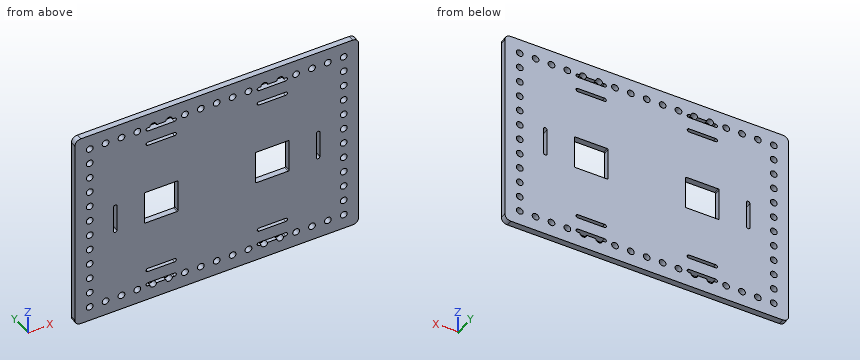
```python
from build123d import *

# Parameters (mm, degrees)
SKETCH1_R           = 1.7
BOSS_EXTRUDE1_DEPTH = 3


with BuildPart() as part:
    # Sketch1 → Boss-Extrude1 (new body)
    with BuildSketch(Plane(origin=(0, 3, 0), x_dir=(1, 0, 0), z_dir=(0, 1, 0))):
        with BuildLine():
            Line((71.5, -48.5), (71.5, 48.5))
            ThreePointArc((71.5, 48.5), (70.621320344, 50.621320344), (68.5, 51.5))
            Line((68.5, 51.5), (-68.5, 51.5))
            ThreePointArc((-68.5, 51.5), (-70.621320344, 50.621320344), (-71.5, 48.5))
            Line((-71.5, 48.5), (-71.5, -48.5))
            ThreePointArc((-71.5, -48.5), (-70.621320344, -50.621320344), (-68.5, -51.5))
            Line((-68.5, -51.5), (68.5, -51.5))
            ThreePointArc((68.5, -51.5), (70.621320344, -50.621320344), (71.5, -48.5))
        make_face()
        with Locations(Location((-64, 44, 0), (0, 0, 90))):
            Circle(SKETCH1_R, mode=Mode.SUBTRACT)
        with Locations(Location((-64, 28, 0), (0, 0, 90))):
            Circle(SKETCH1_R, mode=Mode.SUBTRACT)
        with Locations(Location((-64, 12, 0), (0, 0, 90))):
            Circle(SKETCH1_R, mode=Mode.SUBTRACT)
        with Locations(Location((-64, -4, 0), (0, 0, 90))):
            Circle(SKETCH1_R, mode=Mode.SUBTRACT)
        with Locations(Location((-64, -20, 0), (0, 0, 90))):
            Circle(SKETCH1_R, mode=Mode.SUBTRACT)
        with Locations(Location((-64, -36, 0), (0, 0, 90))):
            Circle(SKETCH1_R, mode=Mode.SUBTRACT)
        with Locations(Location((56, -44, 0), (0, 0, 90))):
            Circle(SKETCH1_R, mode=Mode.SUBTRACT)
        with Locations(Location((40, -44, 0), (0, 0, 90))):
            Circle(SKETCH1_R, mode=Mode.SUBTRACT)
        with Locations(Location((8, -44, 0), (0, 0, 90))):
            Circle(SKETCH1_R, mode=Mode.SUBTRACT)
        with Locations(Location((-8, -44, 0), (0, 0, 90))):
            Circle(SKETCH1_R, mode=Mode.SUBTRACT)
        with Locations(Location((-40, -44, 0), (0, 0, 90))):
            Circle(SKETCH1_R, mode=Mode.SUBTRACT)
        with Locations(Location((-56, -44, 0), (0, 0, 90))):
            Circle(SKETCH1_R, mode=Mode.SUBTRACT)
        with Locations(Location((-64, -44, 0), (0, 0, 90))):
            Circle(SKETCH1_R, mode=Mode.SUBTRACT)
        with Locations(Location((-48, -44, 0), (0, 0, 90))):
            Circle(SKETCH1_R, mode=Mode.SUBTRACT)
        with Locations(Location((-16, -44, 0), (0, 0, 90))):
            Circle(SKETCH1_R, mode=Mode.SUBTRACT)
        with Locations(Location((0, -44, 0), (0, 0, 90))):
            Circle(SKETCH1_R, mode=Mode.SUBTRACT)
        with Locations(Location((16, -44, 0), (0, 0, 90))):
            Circle(SKETCH1_R, mode=Mode.SUBTRACT)
        with Locations(Location((48, -44, 0), (0, 0, 90))):
            Circle(SKETCH1_R, mode=Mode.SUBTRACT)
        with Locations(Location((64, -44, 0), (0, 0, 90))):
            Circle(SKETCH1_R, mode=Mode.SUBTRACT)
        with Locations(Location((-64, -28, 0), (0, 0, 90))):
            Circle(SKETCH1_R, mode=Mode.SUBTRACT)
        with Locations(Location((-64, -12, 0), (0, 0, 90))):
            Circle(SKETCH1_R, mode=Mode.SUBTRACT)
        with Locations(Location((-64, 4, 0), (0, 0, 90))):
            Circle(SKETCH1_R, mode=Mode.SUBTRACT)
        with Locations(Location((-64, 20, 0), (0, 0, 90))):
            Circle(SKETCH1_R, mode=Mode.SUBTRACT)
        with Locations(Location((-64, 36, 0), (0, 0, 90))):
            Circle(SKETCH1_R, mode=Mode.SUBTRACT)
        with Locations(Location((64, -20, 0), (0, 0, 90))):
            Circle(SKETCH1_R, mode=Mode.SUBTRACT)
        with Locations(Location((64, -4, 0), (0, 0, 90))):
            Circle(SKETCH1_R, mode=Mode.SUBTRACT)
        with Locations(Location((64, 12, 0), (0, 0, 90))):
            Circle(SKETCH1_R, mode=Mode.SUBTRACT)
        with Locations(Location((64, 28, 0), (0, 0, 90))):
            Circle(SKETCH1_R, mode=Mode.SUBTRACT)
        with Locations(Location((-48, 44, 0), (0, 0, 90))):
            Circle(SKETCH1_R, mode=Mode.SUBTRACT)
        with Locations(Location((-16, 44, 0), (0, 0, 90))):
            Circle(SKETCH1_R, mode=Mode.SUBTRACT)
        with Locations(Location((0, 44, 0), (0, 0, 90))):
            Circle(SKETCH1_R, mode=Mode.SUBTRACT)
        with Locations(Location((16, 44, 0), (0, 0, 90))):
            Circle(SKETCH1_R, mode=Mode.SUBTRACT)
        with Locations(Location((48, 44, 0), (0, 0, 90))):
            Circle(SKETCH1_R, mode=Mode.SUBTRACT)
        with Locations(Location((64, 44, 0), (0, 0, 90))):
            Circle(SKETCH1_R, mode=Mode.SUBTRACT)
        with Locations(Location((56, 44, 0), (0, 0, 90))):
            Circle(SKETCH1_R, mode=Mode.SUBTRACT)
        with Locations(Location((40, 44, 0), (0, 0, 90))):
            Circle(SKETCH1_R, mode=Mode.SUBTRACT)
        with Locations(Location((8, 44, 0), (0, 0, 90))):
            Circle(SKETCH1_R, mode=Mode.SUBTRACT)
        with Locations(Location((-8, 44, 0), (0, 0, 90))):
            Circle(SKETCH1_R, mode=Mode.SUBTRACT)
        with Locations(Location((-40, 44, 0), (0, 0, 90))):
            Circle(SKETCH1_R, mode=Mode.SUBTRACT)
        with Locations(Location((-56, 44, 0), (0, 0, 90))):
            Circle(SKETCH1_R, mode=Mode.SUBTRACT)
        with Locations(Location((64, 36, 0), (0, 0, 90))):
            Circle(SKETCH1_R, mode=Mode.SUBTRACT)
        with Locations(Location((64, 20, 0), (0, 0, 90))):
            Circle(SKETCH1_R, mode=Mode.SUBTRACT)
        with Locations(Location((64, 4, 0), (0, 0, 90))):
            Circle(SKETCH1_R, mode=Mode.SUBTRACT)
        with Locations(Location((64, -12, 0), (0, 0, 90))):
            Circle(SKETCH1_R, mode=Mode.SUBTRACT)
        with Locations(Location((64, -28, 0), (0, 0, 90))):
            Circle(SKETCH1_R, mode=Mode.SUBTRACT)
        with Locations(Location((64, -36, 0), (0, 0, 90))):
            Circle(SKETCH1_R, mode=Mode.SUBTRACT)
        with BuildLine():
            Line((21.25, 44.05), (22.300735453, 44.05))
            ThreePointArc((22.300735453, 44.05), (24, 45.7), (25.699264547, 44.05))
            Line((25.699264547, 44.05), (30.300735453, 44.05))
            ThreePointArc((30.300735453, 44.05), (32, 45.7), (33.699264547, 44.05))
            Line((33.699264547, 44.05), (34.75, 44.05))
            ThreePointArc((34.75, 44.05), (35.625, 43.175), (34.75, 42.3))
            Line((34.75, 42.3), (21.25, 42.3))
            ThreePointArc((21.25, 42.3), (20.375, 43.175), (21.25, 44.05))
        make_face(mode=Mode.SUBTRACT)
        with BuildLine():
            Line((22.300735453, -44.05), (21.25, -44.05))
            ThreePointArc((21.25, -44.05), (20.375, -43.175), (21.25, -42.3))
            Line((21.25, -42.3), (34.75, -42.3))
            ThreePointArc((34.75, -42.3), (35.625, -43.175), (34.75, -44.05))
            Line((34.75, -44.05), (33.699264547, -44.05))
            ThreePointArc((33.699264547, -44.05), (32, -45.7), (30.300735453, -44.05))
            Line((30.300735453, -44.05), (25.699264547, -44.05))
            ThreePointArc((25.699264547, -44.05), (24, -45.7), (22.300735453, -44.05))
        make_face(mode=Mode.SUBTRACT)
        with BuildLine():
            Line((21.25, 36.05), (34.75, 36.05))
            ThreePointArc((34.75, 36.05), (35.625, 35.175), (34.75, 34.3))
            Line((34.75, 34.3), (21.25, 34.3))
            ThreePointArc((21.25, 34.3), (20.375, 35.175), (21.25, 36.05))
        make_face(mode=Mode.SUBTRACT)
        with BuildLine():
            Line((50.25, -6.75), (50.25, 6.75))
            ThreePointArc((50.25, 6.75), (51.125, 7.625), (52, 6.75))
            Line((52, 6.75), (52, -6.75))
            ThreePointArc((52, -6.75), (51.125, -7.625), (50.25, -6.75))
        make_face(mode=Mode.SUBTRACT)
        with BuildLine():
            Line((21.25, -34.3), (34.75, -34.3))
            ThreePointArc((34.75, -34.3), (35.625, -35.175), (34.75, -36.05))
            Line((34.75, -36.05), (21.25, -36.05))
            ThreePointArc((21.25, -36.05), (20.375, -35.175), (21.25, -34.3))
        make_face(mode=Mode.SUBTRACT)
        with BuildLine():
            Line((36, -8.5), (20, -8.5))
            ThreePointArc((20, -8.5), (19.646446609, -8.353553391), (19.5, -8))
            Line((19.5, -8), (19.5, 8))
            ThreePointArc((19.5, 8), (19.646446609, 8.353553391), (20, 8.5))
            Line((20, 8.5), (36, 8.5))
            ThreePointArc((36, 8.5), (36.353553391, 8.353553391), (36.5, 8))
            Line((36.5, 8), (36.5, -8))
            ThreePointArc((36.5, -8), (36.353553391, -8.353553391), (36, -8.5))
        make_face(mode=Mode.SUBTRACT)
        with BuildLine():
            Line((-21.25, 34.3), (-34.75, 34.3))
            ThreePointArc((-34.75, 34.3), (-35.625, 35.175), (-34.75, 36.05))
            Line((-34.75, 36.05), (-21.25, 36.05))
            ThreePointArc((-21.25, 36.05), (-20.375, 35.175), (-21.25, 34.3))
        make_face(mode=Mode.SUBTRACT)
        with BuildLine():
            Line((-50.25, 6.75), (-50.25, -6.75))
            ThreePointArc((-50.25, -6.75), (-51.125, -7.625), (-52, -6.75))
            Line((-52, -6.75), (-52, 6.75))
            ThreePointArc((-52, 6.75), (-51.125, 7.625), (-50.25, 6.75))
        make_face(mode=Mode.SUBTRACT)
        with BuildLine():
            Line((-21.25, -36.05), (-34.75, -36.05))
            ThreePointArc((-34.75, -36.05), (-35.625, -35.175), (-34.75, -34.3))
            Line((-34.75, -34.3), (-21.25, -34.3))
            ThreePointArc((-21.25, -34.3), (-20.375, -35.175), (-21.25, -36.05))
        make_face(mode=Mode.SUBTRACT)
        with BuildLine():
            Line((-19.5, 8), (-19.5, -8))
            ThreePointArc((-19.5, -8), (-19.646446609, -8.353553391), (-20, -8.5))
            Line((-20, -8.5), (-36, -8.5))
            ThreePointArc((-36, -8.5), (-36.353553391, -8.353553391), (-36.5, -8))
            Line((-36.5, -8), (-36.5, 8))
            ThreePointArc((-36.5, 8), (-36.353553391, 8.353553391), (-36, 8.5))
            Line((-36, 8.5), (-20, 8.5))
            ThreePointArc((-20, 8.5), (-19.646446609, 8.353553391), (-19.5, 8))
        make_face(mode=Mode.SUBTRACT)
        with BuildLine():
            Line((-34.75, -42.3), (-21.25, -42.3))
            ThreePointArc((-21.25, -42.3), (-20.375, -43.175), (-21.25, -44.05))
            Line((-21.25, -44.05), (-22.300735453, -44.05))
            ThreePointArc((-22.300735453, -44.05), (-24, -45.7), (-25.699264547, -44.05))
            Line((-25.699264547, -44.05), (-30.300735453, -44.05))
            ThreePointArc((-30.300735453, -44.05), (-32, -45.7), (-33.699264547, -44.05))
            Line((-33.699264547, -44.05), (-34.75, -44.05))
            ThreePointArc((-34.75, -44.05), (-35.625, -43.175), (-34.75, -42.3))
        make_face(mode=Mode.SUBTRACT)
        with BuildLine():
            Line((-34.75, 44.05), (-33.699264547, 44.05))
            ThreePointArc((-33.699264547, 44.05), (-32, 45.7), (-30.300735453, 44.05))
            Line((-30.300735453, 44.05), (-25.699264547, 44.05))
            ThreePointArc((-25.699264547, 44.05), (-24, 45.7), (-22.300735453, 44.05))
            Line((-22.300735453, 44.05), (-21.25, 44.05))
            ThreePointArc((-21.25, 44.05), (-20.375, 43.175), (-21.25, 42.3))
            Line((-21.25, 42.3), (-34.75, 42.3))
            ThreePointArc((-34.75, 42.3), (-35.625, 43.175), (-34.75, 44.05))
        make_face(mode=Mode.SUBTRACT)
    extrude(amount=-BOSS_EXTRUDE1_DEPTH)


solid = part.part
```
Build history of the part. All positions in model axes, mm. Give positions to 0.01 mm unless a question says otherwise; leave off trailing zeros. Loops run counter-clockwise (first coordinate to the right, second up) from the corner with the lowest first, then second, coordinate; pieces in that order, holes last.
1) Drop a flat-ended pin along its axis: P1, Ø4.5, axis at x = -48, z = -44, coming from the -Y side. Give the stop position or say it passes through.
Values follow:
P1: stops at y = 0
2) Probe line 1 along X through (y, z) = (0.7, -12); line 2 along Z through (x, y) = (-48, 2.35); line 3 along Z through (x, y) = (30, 1.95). List the from-to ranges inside material, lowest first.
Values follow:
line 1: x = -71.5 to -65.7, -62.3 to 62.3, 65.7 to 71.5
line 2: z = -51.5 to -45.7, -42.3 to 42.3, 45.7 to 51.5
line 3: z = -51.5 to -44.05, -42.3 to -36.05, -34.3 to -8.5, 8.5 to 34.3, 36.05 to 42.3, 44.05 to 51.5
3) Band-saw the part on D-D on x = -64. State how many separate pieces and enclosed holes the cut face has, then the cut area to 3 significant figures.
Values follow:
separate pieces: 13
enclosed holes: 0
area: 187 mm2
4) Band-saw the part on C-C on x = -32. List the corners of the cut face in (y, z), then the cut area to 3 significant figures.
Values follow:
outline: (0, -51.5) - (3, -51.5) - (3, -45.7) - (0, -45.7) - close; (0, -42.3) - (3, -42.3) - (3, -36.05) - (0, -36.05) - close; (0, -34.3) - (3, -34.3) - (3, -8.5) - (0, -8.5) - close; (0, 8.5) - (3, 8.5) - (3, 34.3) - (0, 34.3) - close; (0, 36.05) - (3, 36.05) - (3, 42.3) - (0, 42.3) - close; (0, 45.7) - (3, 45.7) - (3, 51.5) - (0, 51.5) - close
area: 227 mm2
5) Band-saw the part on B-B on z = -20. List the corners of the cut face in (x, y), then the cut area to 3 significant figures.
Values follow:
outline: (-71.5, 0) - (-65.7, 0) - (-65.7, 3) - (-71.5, 3) - close; (-62.3, 0) - (62.3, 0) - (62.3, 3) - (-62.3, 3) - close; (65.7, 0) - (71.5, 0) - (71.5, 3) - (65.7, 3) - close
area: 409 mm2
6) Band-saw the part on A-A on x = -8. List the corners of the cut face in (y, z), then the cut area to 3 significant figures.
Values follow:
outline: (0, -51.5) - (3, -51.5) - (3, -45.7) - (0, -45.7) - close; (0, -42.3) - (3, -42.3) - (3, 42.3) - (0, 42.3) - close; (0, 45.7) - (3, 45.7) - (3, 51.5) - (0, 51.5) - close
area: 289 mm2
